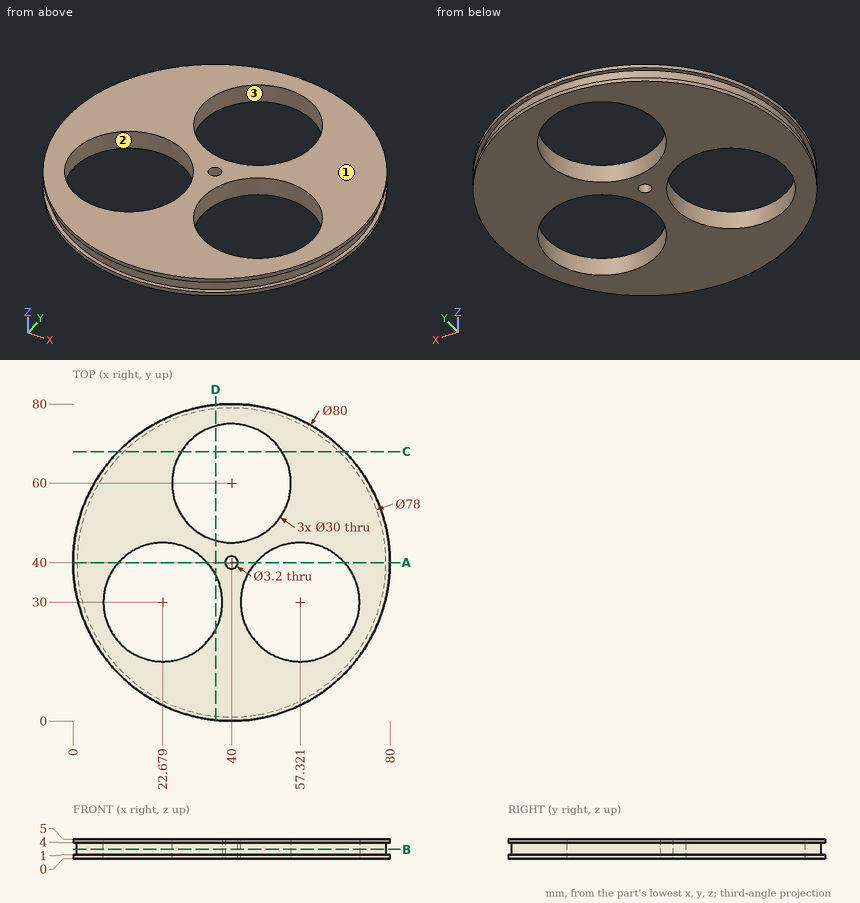
Job drawing, mm, ordinate dimensions from the low corner. One solid piece. Coordinates: 2 decimals unless noted, no trailing zeros. Write each loop counter-clockwise with the first axis right and the second up, starting at its lowest first coordinate (ties: lowest second). Pieces come first, ordered by that corner, then holes. Notation, with made-up numbers: M 60,81 L 101,81 A27 ccw 101,106 Z; hole C 52.25,56 d7. An arc over 180 degrees is marked long. Answer as a JSON object with one key per item and string values. Group by question number.
1) Saw through at C-C (y = 68). Write the cut outline in (x, z) (1 decimal).
2) Wall check: line 1 (Y direction, x = 40, z = 2.8); line 2 (X direction, y = 40.5, z = 3.15) (1 decimal); line 3 (X direction, y = 43, z = 2.45) (1 decimal). Give the ranges that are in metal, low to high. Write a range as from..to.
3) Pin check, flat tips, straight feed: pin 1 Ø1.5 at (x, z) = (63.5, 2.5) entering from -Y; pin 2 Ø1 at (x, z) = (53, 0.5) entering from +Y. Stop position of each tip, or through.
4) Mould opens along Y. For the marked faces 1, 2 and 3 say: +Y half, -Y half, draft (parallel to the pull), parting line (faces both ways), or undercut.
5) Saw through at D-D (x = 36). Write the cut outline in (y, z) (1 decimal).
6) Saw through at B-B (z = 2.4). Write the cut outline in (x, y), plus the area to 3 significant figures.
7) Saw through at A-A (y = 40). Write the cut outline in (x, z).
Values follow:
{
 "1": {"outline": "M 11.4,0 L 27.3,0 L 27.3,5 L 11.4,5 L 11.4,4 L 12.9,4 L 12.9,1 L 11.4,1 Z; M 52.7,0 L 68.6,0 L 68.6,1 L 67.1,1 L 67.1,4 L 68.6,4 L 68.6,5 L 52.7,5 Z"},
 "2": {"line 1": "y = 1..38.4, 41.6..45, 75..79", "line 2": "x = 1..12, 33.4..38.5, 41.5..46.6, 68..79", "line 3": "x = 1.1..15.2, 30.2..49.8, 64.8..78.9"},
 "3": {"pin 1": "stops at y = 8.32", "pin 2": "stops at y = 78"},
 "4": {"face 1": "draft", "face 2": "undercut", "face 3": "undercut"},
 "5": {"outline": "M 0.2,0 L 23.1,0 L 23.1,5 L 0.2,5 L 0.2,4 L 1.2,4 L 1.2,1 L 0.2,1 Z; M 36.9,0 L 45.5,0 L 45.5,5 L 36.9,5 Z; M 74.5,0 L 79.8,0 L 79.8,1 L 78.8,1 L 78.8,4 L 79.8,4 L 79.8,5 L 74.5,5 Z"},
 "6": {"outline": "C 40,40 d78; hole C 22.68,30 d30; hole C 40,60 d30; hole C 40,40 d3.2; hole C 57.32,30 d30", "area": "2,650 mm2"},
 "7": {"outline": "M 0,0 L 11.5,0 L 11.5,5 L 0,5 L 0,4 L 1,4 L 1,1 L 0,1 Z; M 33.86,0 L 38.4,0 L 38.4,5 L 33.86,5 Z; M 41.6,0 L 46.14,0 L 46.14,5 L 41.6,5 Z; M 68.5,0 L 80,0 L 80,1 L 79,1 L 79,4 L 80,4 L 80,5 L 68.5,5 Z"}
}
